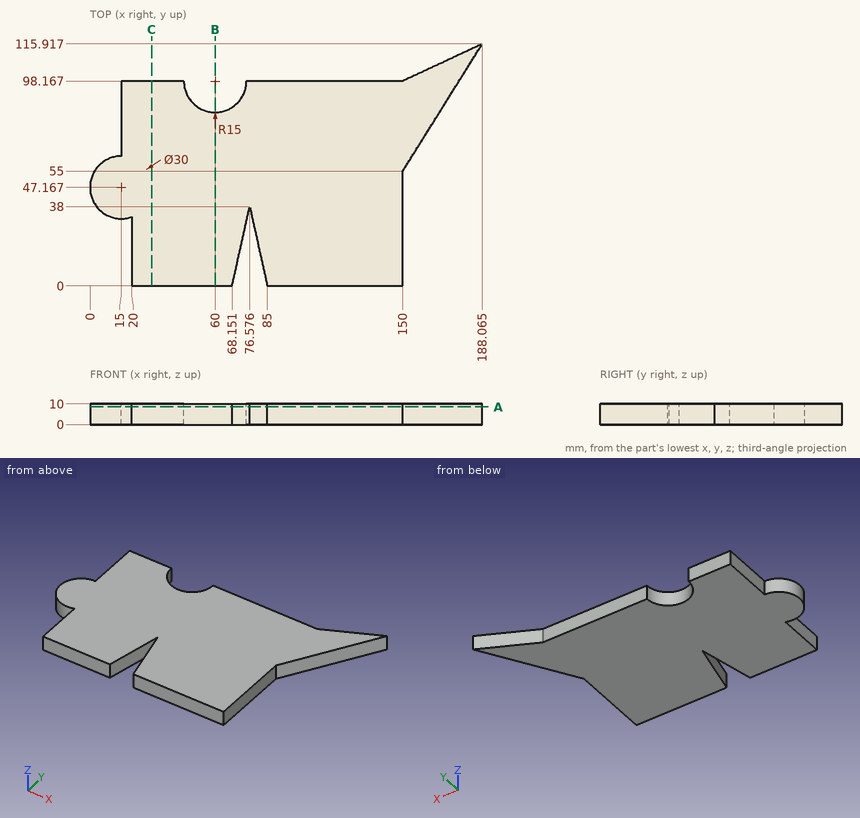
The figure shows three views and two pictorial views of one solid part (mm, origin at its lowest corner). Answer the questions. Give positions to 0.01 mm unless a question says otherwise; leave off trailing zeros. Write each loop counter-clockwise with the first axis right and the second up, starting at its lowest first coordinate (ties: lowest second). Pieces come first, ordered by that corner, then holes. Notation, with made-up numbers: (36, 64) - (75, 64) arc R27 cw to (75, 98) - close; hole circle Ø6 at (83, -18). An arc over 180 degrees is marked (long way). Use CSV: the item, a comma, the result in double quotes. Start each with the question number.
Item 1: The part is cut by section A-A, the plane z = 8.5. Give the vertices of the cut face in (x, y) (1 decimal).
Item 2: The part is cut by section B-B, the plane x = 60. Give the vertices of the cut face in (y, z).
Item 3: The part is cut by section C-C, the plane x = 29.5. Give the vertices of the cut face in (y, z).
Item 4: Flat-ended cylindrical pins translate along their axes: P1, Ø1.5, axis at x = 158.5, z = 4.5, coming from the +Y side; P2, Ø8, axis at x = 156.5, y = 17.5, coming from the +Z side; P3, Ø2, axis at x = 33.5, z = 2.5, coming from the +Y side; P4, Ø5, axis at y = 26, z = 5, coming from the +X side. Find the tip coordinate at first contact, or state that the pin passes through.
Item 5: Consider line 1 (X direction, y = 20, z = 8.75) (1 decimal); line 2 (Y direction, x = 43, z = 7.75); line 3 (X direction, y = 18.5, z = 5.75). Determine where each line is inside the solid, lowest interval first.
Taken from the geometry:
1,outline,"(15, 62.2) arc R15 ccw (long way) to (20, 33) - (20, 0) - (68.2, 0) - (76.6, 38) - (85, 0) - (150, 0) - (150, 55) - (188.1, 115.9) - (150, 98.2) - (75, 98.2) arc R15 cw to (45, 98.2) - (15, 98.2) - close"
2,outline,"(0, 0) - (83.17, 0) - (83.17, 10) - (0, 10) - close"
3,outline,"(0, 0) - (98.17, 0) - (98.17, 10) - (0, 10) - close"
4,P1,"y = 102.48"
4,P2,"through"
4,P3,"y = 98.17"
4,P4,"x = 150"
5,line 1,"20 to 72.6, 80.6 to 150"
5,line 2,"0 to 98.17"
5,line 3,"20 to 72.25, 80.9 to 150"
